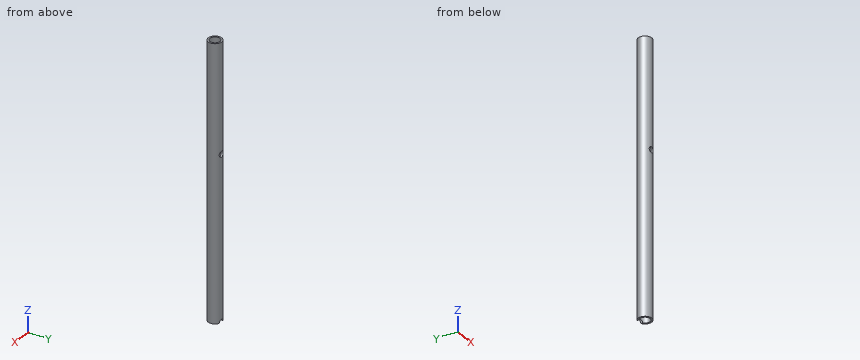
Autodesk Fusion 360 part; units mm, degrees
sketch "Esquisse1" plane through (0, 0, 0) normal (0, 0, 1) x (1, 0, 0)
  circle A0 centre (0, 0) radius 4
  circle A1 centre (0, 0) radius 3
  dimension "d1" = 8
  dimension "d2" = 6
extrude "Extrusion1" add sketch "Esquisse1" along normal blind 160
hole "Perçage1" at (0, 0, 0) direction (0, 1, 0) diameter 3.5 depth 8 tip angle 180
hole "Perçage2" at (0, 4, 96) direction (0, -1, 0) diameter 3.5 depth 8 tip angle 180
Geometry check sheet. Reference: the model listing, model coordinates, mm. Round coordinates to 2 decimals unless told otherwise and drop trailing zeros. Loops run counter-clockwise (first coordinate to the right, second up) from the corner with the lowest first, then second, coordinate; pieces in that order, holes last. Notation, with made-up numbers: (72, 76) - (110, 76) arc R30 cw to (110, 105) - close; hole circle Ø5 at (38.5, -20.75). An arc over 180 degrees is marked (long way). Write item = value, one per line. Start each with the question number.
1. Thickness scan on line 1 (Z direction, x = 0, y = 3.15); line 2 (Y direction, x = 0, z = 101.5). Record the ranges inside material, lowest first.
2. Section check D-D on z = 23. Enter the section's corners in (x, y), then the cut area to 3 significant figures.
3. Depth check by flat-ended pin: pin 1 (3 mm diameter, centred on y = -2, z = 82.5, fed in from +X); pin 2 (1 mm diameter, centred on x = -0.5, y = 1.5, fed in from -Z); pin 3 (1.5 mm diameter, centred on x = -1, z = 65.5, fed in from +Y). Enter the tip coordinate at first touch or a pass-through.
4. Section check A-A on x = 0. Enter the section's corners in (y, z).
5. Section check C-C on z = 96. Enter the section's corners in (x, y).
6. Section check B-B on y = 0. Enter the section's corners in (x, z), then the cut area to 3 significant figures.
Working result:
q1.line_1 = 1.75 to 94.25, 97.75 to 160
q1.line_2 = -4 to -3, 3 to 4
q2.outline = circle Ø8 at (0, 0); hole circle Ø6 at (0, 0)
q2.area = 22.0 mm^2
q3.pin_1 = 3.97
q3.pin_2 = through
q3.pin_3 = 3.99
q4.outline = (-4, 0) - (-3, 0) - (-3, 94.25) - (-4, 94.25) - close; (-4, 97.75) - (-3, 97.75) - (-3, 160) - (-4, 160) - close; (3, 1.75) - (4, 1.75) - (4, 94.25) - (3, 94.25) - close; (3, 97.75) - (4, 97.75) - (4, 160) - (3, 160) - close
q5.outline = (-1.75, -3.6) - (-1.75, -2.44) arc R3 cw to (-1.75, 2.44) - (-1.75, 3.6) arc R4 ccw to start; (1.75, -3.6) arc R4 ccw to (1.75, 3.6) - (1.75, 2.44) arc R3 cw to (1.75, -2.44) - close
q6.outline = (-4, 0) - (-3, 0) - (-3, 160) - (-4, 160) - close; (3, 0) - (4, 0) - (4, 160) - (3, 160) - close
q6.area = 320 mm^2
